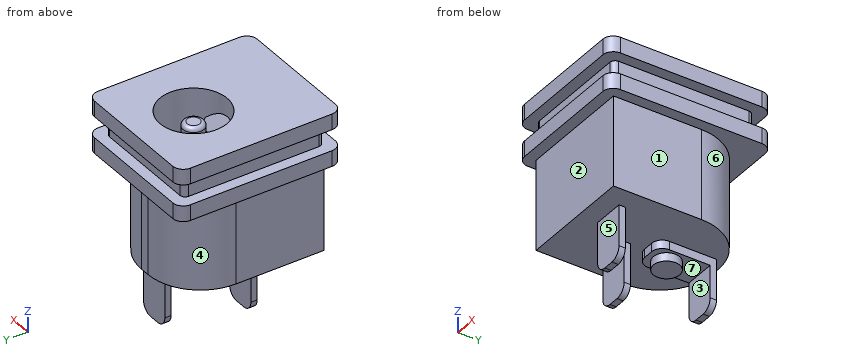
from build123d import *

# Parameters (mm, degrees)
EXTRUDE_1_DEPTH     = 1.5
EXTRUDE_2_DEPTH     = 2
EXTRUDE_START       = 1.5
EXTRUDE_3_DEPTH     = 1.5
EXTRUDE_4_DEPTH     = 8.6
SKETCH_5_R          = 3.2
CUT_EXTRUDE_1_DEPTH = 10
SKETCH_6_R          = 1
EXTRUDE_5_DEPTH     = 9
FILLET_1_R          = 0.4
SKETCH_8_W          = 4
SKETCH_8_H          = 0.3
SKETCH_11_W         = 3
SKETCH_11_H         = 0.6
EXTRUDE_6_DEPTH     = 4.9
SKETCH_12_W         = 3
SKETCH_12_H         = 5.5
EXTRUDE_7_DEPTH     = 0.8
SKETCH_13_R         = 1.25
EXTRUDE_8_DEPTH     = 1.6
FILLET_2_R          = 1
FILLET_3_R          = 1


with BuildPart() as part:
    # Эскиз1 → Бобышка-Вытянуть1 (new body)
    with BuildSketch(Plane.XY):
        with BuildLine():
            Line((5.5, -7.75), (-5.5, -7.75))
            ThreePointArc((-5.5, -7.75), (-6.207106781, -7.457106781), (-6.5, -6.75))
            Line((-6.5, -6.75), (-6.5, 6.75))
            ThreePointArc((-6.5, 6.75), (-6.207106781, 7.457106781), (-5.5, 7.75))
            Line((-5.5, 7.75), (5.5, 7.75))
            ThreePointArc((5.5, 7.75), (6.207106781, 7.457106781), (6.5, 6.75))
            Line((6.5, 6.75), (6.5, -6.75))
            ThreePointArc((6.5, -6.75), (6.207106781, -7.457106781), (5.5, -7.75))
        make_face()
    extrude(amount=EXTRUDE_1_DEPTH)

    # Эскиз2 → Бобышка-Вытянуть2 (add)
    with BuildSketch(Plane.XY):
        with BuildLine():
            Line((4.95, -6.7), (-4.95, -6.7))
            ThreePointArc((-4.95, -6.7), (-5.303553391, -6.553553391), (-5.45, -6.2))
            Line((-5.45, -6.2), (-5.45, 6.2))
            ThreePointArc((-5.45, 6.2), (-5.303553391, 6.553553391), (-4.95, 6.7))
            Line((-4.95, 6.7), (4.95, 6.7))
            ThreePointArc((4.95, 6.7), (5.303553391, 6.553553391), (5.45, 6.2))
            Line((5.45, 6.2), (5.45, -6.2))
            ThreePointArc((5.45, -6.2), (5.303553391, -6.553553391), (4.95, -6.7))
        make_face()
    extrude(amount=-EXTRUDE_2_DEPTH)

    # Эскиз3 → Бобышка-Вытянуть3 (add)
    with BuildSketch(Plane(origin=(0, 0, -2), x_dir=(-1, 0, 0), z_dir=(0, 0, -1)).offset(EXTRUDE_START)):
        with BuildLine():
            Line((-5.5, -7.75), (5.5, -7.75))
            ThreePointArc((5.5, -7.75), (6.207106781, -7.457106781), (6.5, -6.75))
            Line((6.5, -6.75), (6.5, 6.75))
            ThreePointArc((6.5, 6.75), (6.207106781, 7.457106781), (5.5, 7.75))
            Line((5.5, 7.75), (-5.5, 7.75))
            ThreePointArc((-5.5, 7.75), (-6.207106781, 7.457106781), (-6.5, 6.75))
            Line((-6.5, 6.75), (-6.5, -6.75))
            ThreePointArc((-6.5, -6.75), (-6.207106781, -7.457106781), (-5.5, -7.75))
        make_face()
    extrude(amount=-EXTRUDE_3_DEPTH)

    # Эскиз4 → Бобышка-Вытянуть4 (add)
    with BuildSketch(Plane(origin=(0, 0, -3.5), x_dir=(-1, 0, 0), z_dir=(0, 0, -1))):
        with BuildLine():
            Line((-5.45, -6.7), (5.45, -6.7))
            Line((5.45, -6.7), (5.45, 1.7))
            ThreePointArc((5.45, 1.7), (3.985533906, 5.235533906), (0.45, 6.7))
            Line((0.45, 6.7), (-0.45, 6.7))
            ThreePointArc((-0.45, 6.7), (-3.985533906, 5.235533906), (-5.45, 1.7))
            Line((-5.45, 1.7), (-5.45, -6.7))
        make_face()
    extrude(amount=EXTRUDE_4_DEPTH)

    # Эскиз5 → Вырез-Вытянуть1 (cut)
    with BuildSketch(Plane.XY.offset(1.5)):
        with Locations((0, 2.05)):
            Circle(SKETCH_5_R)
    extrude(amount=-CUT_EXTRUDE_1_DEPTH, mode=Mode.SUBTRACT)

    # Эскиз6 → Бобышка-Вытянуть5 (add)
    with BuildSketch(Plane.XY.offset(-8.5)):
        with Locations((0, 2.05)):
            Circle(SKETCH_6_R)
    extrude(amount=EXTRUDE_5_DEPTH)

    # Скругление1
    fillet_1_edges = [part.edges().sort_by_distance(p)[0] for p in [
        (-1, 2.05, 0.5),
    ]]
    fillet(fillet_1_edges, radius=FILLET_1_R)

    # По траектории1: sweep along a path in Эскиз9
    with BuildLine(Plane(origin=(0, 0, 0), x_dir=(0, 0, -1), z_dir=(1, 0, 0))) as sweep_1_path:
        Line((0, -1.5), (1.866666667, -0.1))
        ThreePointArc((1.866666667, -0.1), (2.008552784, -0.025658351), (2.166666667, 0))
        Line((2.166666667, 0), (2.833333333, 0))
        ThreePointArc((2.833333333, 0), (2.991447216, -0.025658351), (3.133333333, -0.1))
        Line((3.133333333, -0.1), (4.866666667, -1.4))
        ThreePointArc((4.866666667, -1.4), (5.008552784, -1.474341649), (5.166666667, -1.5))
        Line((5.166666667, -1.5), (8.166666667, -1.5))
    # Эскиз8 → По траектории1 (sweep)
    with BuildSketch(Plane.XY):
        with Locations((0, -1.5)):
            Rectangle(SKETCH_8_W, SKETCH_8_H)
    sweep(path=sweep_1_path.line)

    # Эскиз11 → Бобышка-Вытянуть6 (add)
    with BuildSketch(Plane(origin=(0, 0, -12.1), x_dir=(-1, 0, 0), z_dir=(0, 0, -1))):
        with Locations((-2, -4.55)):
            Rectangle(SKETCH_11_W, SKETCH_11_H)
        with Locations((2, -1.35)):
            Rectangle(SKETCH_11_W, SKETCH_11_H)
        with Locations((0, 5.5)):
            Rectangle(SKETCH_11_W, SKETCH_11_H)
    extrude(amount=EXTRUDE_6_DEPTH)

    # Эскиз12 → Бобышка-Вытянуть7 (add)
    with BuildSketch(Plane(origin=(0, 0, -12.1), x_dir=(-1, 0, 0), z_dir=(0, 0, -1))):
        with Locations((0, 3.05)):
            Rectangle(SKETCH_12_W, SKETCH_12_H)
    extrude(amount=EXTRUDE_7_DEPTH)

    # Эскиз13 → Бобышка-Вытянуть8 (add)
    with BuildSketch(Plane(origin=(0, 0, -12.1), x_dir=(-1, 0, 0), z_dir=(0, 0, -1))):
        with Locations((0, 2.05)):
            Circle(SKETCH_13_R)
    extrude(amount=EXTRUDE_8_DEPTH)

    # Скругление2
    fillet_2_edges = [part.edges().sort_by_distance(p)[0] for p in [
        (-1.5, 0.3, -12.5),
        (1.5, 0.3, -12.5),
    ]]
    fillet(fillet_2_edges, radius=FILLET_2_R)

    # Скругление3
    fillet_3_edges = [part.edges().sort_by_distance(p)[0] for p in [
        (-1.5, 5.5, -17),
        (1.5, 5.5, -17),
        (-3.5, -1.35, -17),
        (-0.5, -1.35, -17),
        (0.5, -4.55, -17),
        (3.5, -4.55, -17),
    ]]
    fillet(fillet_3_edges, radius=FILLET_3_R)


solid = part.part
Could you check a few things on this model? Use its own coordinates, in mm. Face numbers are marked on the shaded views. A direction names the side the tool comes from. Round coordinates to 2 decimals unless told otherwise and drop trailing zeros. Write each loop counter-clockwise with the first axis right and the second up, starting at its lowest first coordinate (ties: lowest second). Pieces come first, ordered by that corner, then holes. Notation, with made-up numbers: (7, 33) -> (12, 33) arc R22 cw to (12, 53) -> close; hole circle Ø10 at (30, -3.5). An arc over 180 degrees is marked (long way). Use a Markdown table: item, result.
1. If we section it at C-C (y = -4): List the corners of the cut face in (x, z) for me.
Answer key:
| item | result |
|---|---|
| outline | (-6.5, -3.5) -> (-5.45, -3.5) -> (-5.45, -12.1) -> (5.45, -12.1) -> (5.45, -3.5) -> (6.5, -3.5) -> (6.5, -2) -> (5.45, -2) -> (5.45, 0) -> (6.5, 0) -> (6.5, 1.5) -> (-6.5, 1.5) -> (-6.5, 0) -> (-5.45, 0) -> (-5.45, -2) -> (-6.5, -2) -> close |
2. If we section it at D-D (x = 3.75): List the corners of the cut face in (y, z) for me, then the cut area to 3 significant figures.
Answer key:
| item | result |
|---|---|
| outline | (-7.75, -3.5) -> (-6.7, -3.5) -> (-6.7, -12.1) -> (5.46, -12.1) -> (5.46, -3.5) -> (7.75, -3.5) -> (7.75, -2) -> (6.7, -2) -> (6.7, 0) -> (7.75, 0) -> (7.75, 1.5) -> (-7.75, 1.5) -> (-7.75, 0) -> (-6.7, 0) -> (-6.7, -2) -> (-7.75, -2) -> close |
| area | 178 mm^2 |
3. Which directions (+Z, -Z, +X, -X, +Y, -Y) give clear straight access to the entire face, cutting with the end or side of a thin tool? Please do the marked faces 1, 2, 3 and 4.
Answer key:
| item | result |
|---|---|
| face 1 | -Z, +X, +Y, -Y |
| face 2 | -Z, +X, -X, -Y |
| face 3 | -Z, +X, -X |
| face 4 | -Z, -X, +Y |
4. Please list where these lines run through material, in increasing order: probe 1 along Y at (x, z) = (0, -5); probe 2 along Y at (x, z) = (0, -3.25); probe 3 along X at (y, z) = (1.25, -2.25).
Answer key:
| item | result |
|---|---|
| probe 1 | y = -6.7 to -1.15, 1.05 to 3.05, 5.25 to 6.7 |
| probe 2 | y = -7.75 to -1.15, -0.34 to -0.03, 1.05 to 3.05, 5.25 to 7.75 |
| probe 3 | x = -6.5 to -3.1, -0.6 to 0.6, 3.1 to 6.5 |
5. For pin 1 Ø3 at (y, z) = (4.5, -15) entering from -X; pin 2 Ø0.9 at (x, z) = (0, -12.5) entering from -Y; pin 3 Ø1 at (x, y) = (0, 2) entering from +Z; pin 4 Ø1 at (y, z) = (-3, -14.5) entering from -X, each with a flat end and sliding along its axis, tell me the tip position at first contact or that it passes through.
Answer key:
| item | result |
|---|---|
| pin 1 | stops at x = -1.5 |
| pin 2 | stops at y = -6.7 |
| pin 3 | stops at z = 0.5 |
| pin 4 | passes through |
6. We'd pull the mould along Y, two halves only. Please class the marked faces 5, 6 and 7: +Y half, -Y half, draft (parallel to the pull), parting line (faces both ways), or undercut.
Answer key:
| item | result |
|---|---|
| face 5 | -Y half |
| face 6 | +Y half |
| face 7 | undercut |
7. If we section it at B-B (z = -15): List the corners of the cut face in (x, y) for me.
Answer key:
| item | result |
|---|---|
| outline | (-3.5, -1.65) -> (-0.5, -1.65) -> (-0.5, -1.05) -> (-3.5, -1.05) -> close; (-1.5, 5.2) -> (1.5, 5.2) -> (1.5, 5.8) -> (-1.5, 5.8) -> close; (0.5, -4.85) -> (3.5, -4.85) -> (3.5, -4.25) -> (0.5, -4.25) -> close |
8. If we section it at A-A (z = -5.25): List the corners of the cut face in (x, y) for me.
Answer key:
| item | result |
|---|---|
| outline | (-5.45, -6.7) -> (5.45, -6.7) -> (5.45, 1.7) arc R5 ccw to (0.45, 6.7) -> (-0.45, 6.7) arc R5 ccw to (-5.45, 1.7) -> close; circle Ø2 at (0, 2.05); hole circle Ø6.4 at (0, 2.05) |
